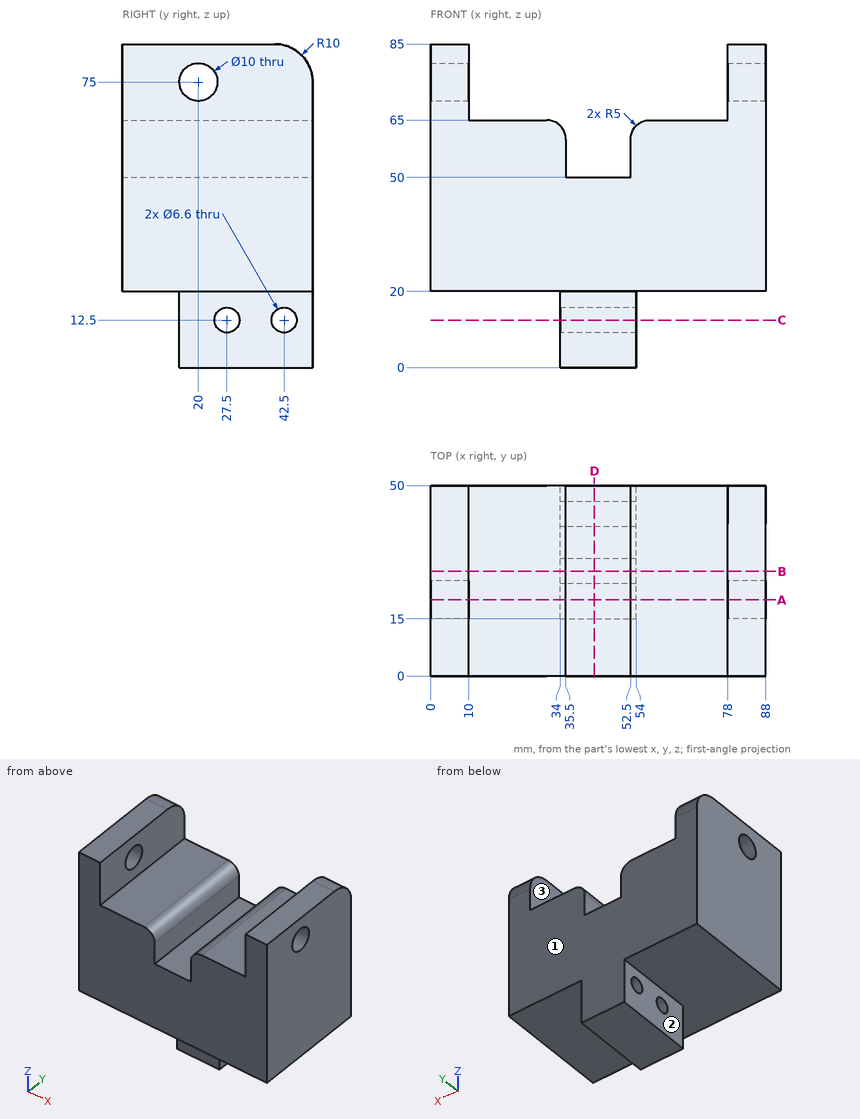
Here's the drawing with two shaded views (mm, measured from the low corner). I have some questions. A direction names the side the tool comes from. Coordinates: 2 decimals unless noted, no trailing zeros. Write each loop counter-clockwise with the first axis right and the second up, starting at its lowest first coordinate (ties: lowest second). Pieces come first, ordered by that corner, then holes.
Item 1: I want a section at A-A on y = 20. Write out the boundary of the cut face in (x, z), and give its area (3 significant figures).
Item 2: I want a section at C-C on z = 12.5. Write out the boundary of the cut face in (x, y).
Item 3: On a 3-axis mill with a long thin cutter (end or side, diameter ignored), from which of +Z, -Z, +X, -X, +Y, -Y can I reach the whole of each face in a straight line? I mean the marked faces 1, 2 and 3. Say none if no direction works.
Item 4: If I drill on line 1 (Y direction, x = 46.5, z = 12.5); line 2 (X direction, y = 36, z = 59.5); line 3 (Z direction, x = 49, y = 48), over which ranges is the centre line in solid material (lowest first)?
Item 5: Will these pins go through, and if not, where does the flat tip stop? pin 1 (1.5 mm diameter, centred on x = 12, y = 29, fed in from +Z); pin 2 (16 mm diameter, centred on x = 39.5, z = 10, fed in from -Y); pin 3 (2 mm diameter, centred on x = 50, y = 18.5, fed in from +Z).
Item 6: I want a section at D-D on x = 43. Write out the boundary of the cut face in (y, z), and give its area (3 significant figures).
Item 7: I want a section at B-B on y = 27.5. Write out the boundary of the cut face in (x, z), and give its area (3 significant figures).
Findings below:
1. outline: (0, 20) - (34, 20) - (34, 0) - (54, 0) - (54, 20) - (88, 20) - (88, 70) - (78, 70) - (78, 65) - (57.5, 65) arc R5 ccw to (52.5, 60) - (52.5, 50) - (35.5, 50) - (35.5, 60) arc R5 ccw to (30.5, 65) - (10, 65) - (10, 70) - (0, 70) - close; (0, 80) - (10, 80) - (10, 85) - (0, 85) - close; (78, 80) - (88, 80) - (88, 85) - (78, 85) - close
1. area: 4,290 mm2
2. outline: (34, 15) - (54, 15) - (54, 24.2) - (34, 24.2) - close; (34, 30.8) - (54, 30.8) - (54, 39.2) - (34, 39.2) - close; (34, 45.8) - (54, 45.8) - (54, 50) - (34, 50) - close
3. face 1: +Z, -Z, +X, -X, +Y
3. face 2: -Z, -X, +Y, -Y
3. face 3: +Z, +Y, -Y
4. line 1: y = 15 to 24.2, 30.8 to 39.2, 45.8 to 50
4. line 2: x = 0 to 35.5, 52.5 to 88
4. line 3: z = 0 to 50
5. pin 1: stops at z = 65
5. pin 2: stops at y = 15
5. pin 3: stops at z = 50
6. outline: (0, 20) - (15, 20) - (15, 0) - (50, 0) - (50, 50) - (0, 50) - close; hole circle Ø6.6 at (27.5, 12.5); hole circle Ø6.6 at (42.5, 12.5)
6. area: 2,130 mm2
7. outline: (0, 20) - (34, 20) - (34, 15.8) - (54, 15.8) - (54, 20) - (88, 20) - (88, 85) - (78, 85) - (78, 65) - (57.5, 65) arc R5 ccw to (52.5, 60) - (52.5, 50) - (35.5, 50) - (35.5, 60) arc R5 ccw to (30.5, 65) - (10, 65) - (10, 85) - (0, 85) - close; (34, 0) - (54, 0) - (54, 9.2) - (34, 9.2) - close
7. area: 4,360 mm2
